Job drawing, mm, ordinate dimensions from the low corner. One solid piece. Coordinates: 2 decimals unless noted, no trailing zeros. Write each loop counter-clockwise with the first axis right and the second up, starting at its lowest first coordinate (ties: lowest second). Pieces come first, ordered by that corner, then holes. Notation, with made-up numbers: M 2.5,7 L 26.5,7 A16 ccw 26.5,12 Z; hole C 16.25,38 d7. An arc over 180 degrees is marked long. Answer as CSV lines item,"result". Start each with the question number.
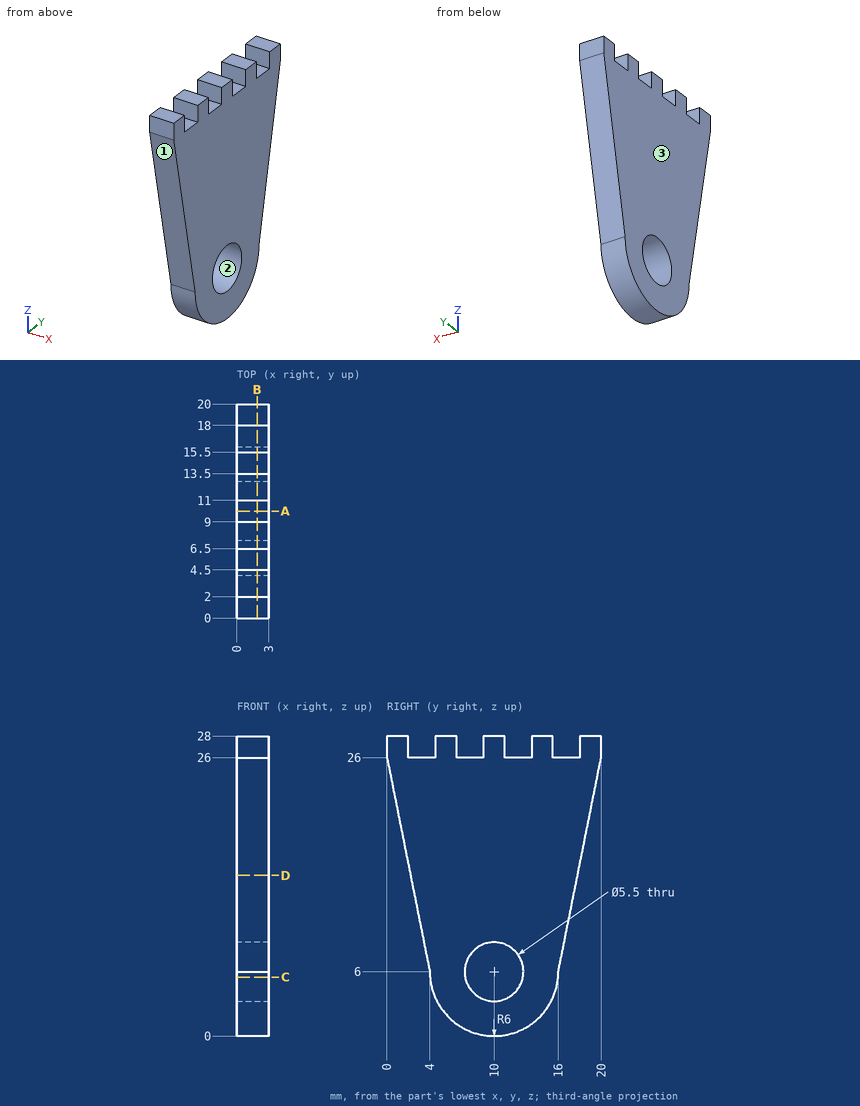
1) Band-saw the part on B-B, the plane x = 1.9. List the corners of the cut face in (y, z).
2) Band-saw the part on D-D, the plane z = 15. List the corners of the cut face in (x, y).
3) Probe L1, parallel to Y at x = 1.55, z = 27.25; L2, parallel to Y at x = 0.8, z = 6; L3, parallel to Z at x = 0.8, y = 7.75. List the from-to ranges inside material, lowest first. Write a range as [from, to].
4) Two-plate mould, pull along Z, no slides. Class the marked faces 1, 2 and 3: pulls with the +Z half, pulls with the -Z half, needs draft (parallel to the pull), parting line crosses it, or undercut.
5) Pin check, flat tips, straight feed: P1, Ø8, axis at y = 3, z = 3.5, coming from the +X side; P2, Ø1.5, axis at x = 1, z = 18, coming from the +Y side; P3, Ø0.8, axis at x = 1, y = 3.5, coming from the +Z side. Stop position of each tip, or through.
6) Band-saw the part on A-A, the plane y = 10. List the corners of the cut face in (x, z), plus the area to 3 significant figures.
7) Band-saw the part on C-C, the plane z = 5.5. List the corners of the cut face in (x, y).
Result sheet:
1,outline,"M 0,26 L 4,6 A6 ccw 16,6 L 20,26 L 20,28 L 18,28 L 18,26 L 15.5,26 L 15.5,28 L 13.5,28 L 13.5,26 L 11,26 L 11,28 L 9,28 L 9,26 L 6.5,26 L 6.5,28 L 4.5,28 L 4.5,26 L 2,26 L 2,28 L 0,28 Z; hole C 10,6 d5.5"
2,outline,"M 0,2.2 L 3,2.2 L 3,17.8 L 0,17.8 Z"
3,L1,"y = [0, 2], [4.5, 6.5], [9, 11], [13.5, 15.5], [18, 20]"
3,L2,"y = [4, 7.25], [12.75, 16]"
3,L3,"z = [0.44, 4.42], [7.58, 26]"
4,face 1,"pulls with the -Z half"
4,face 2,"undercut"
4,face 3,"needs draft"
5,P1,"stops at x = 3"
5,P2,"stops at y = 18.55"
5,P3,"stops at z = 26"
6,outline,"M 0,0 L 3,0 L 3,3.25 L 0,3.25 Z; M 0,8.75 L 3,8.75 L 3,28 L 0,28 Z"
6,area,"67.5 mm²"
7,outline,"M 0,4.02 L 3,4.02 L 3,7.3 L 0,7.3 Z; M 0,12.7 L 3,12.7 L 3,15.98 L 0,15.98 Z"
